Answer from the drawing. Dimensions are ordinates in mm from the lowest x, y and z of the part. Round coordinates to 2 decimals unless told otherwise and drop trailing zeros. Write each loop counter-clockwise with the first axis right and the second up, starting at its lowest first coordinate (ties: lowest second). Pieces come first, ordered by that corner, then holes. Notation, with made-up numbers: M 37.25,10.5 L 81.25,10.5 A27 cw 81.25,28.5 Z; hole C 68.5,43 d5. An arc over 180 degrees is marked long. One line per item, written item: value. Start each with the question number.
(1) Section C-C (z = 1.95) is taken. Determine the outline of the cut face in (x, y).
(2) Section D-D (x = 82.45) is taken. Determine the outline of the cut face in (y, z).
(3) Section A-A (y = 37.5) is taken. Determine the outline of the cut face in (x, z).
(4) Consider probe 1 along Y at (x, z) = (58, 0.8); probe 2 along X at (y, z) = (22, 5.25); probe 3 along Y at (x, z) = (82.45, 1.85). Determine where each line is inside the solid, lowest interval first.
(5) Given P1, Ø3, axis at x = 8.5, z = 2, coming from the -Y side; P2, Ø1.8, axis at x = 13, z = 2, coming from the +Y side, each flat-ended and moving along its own axis, determine where each tip first touches the part or whether it passes through.
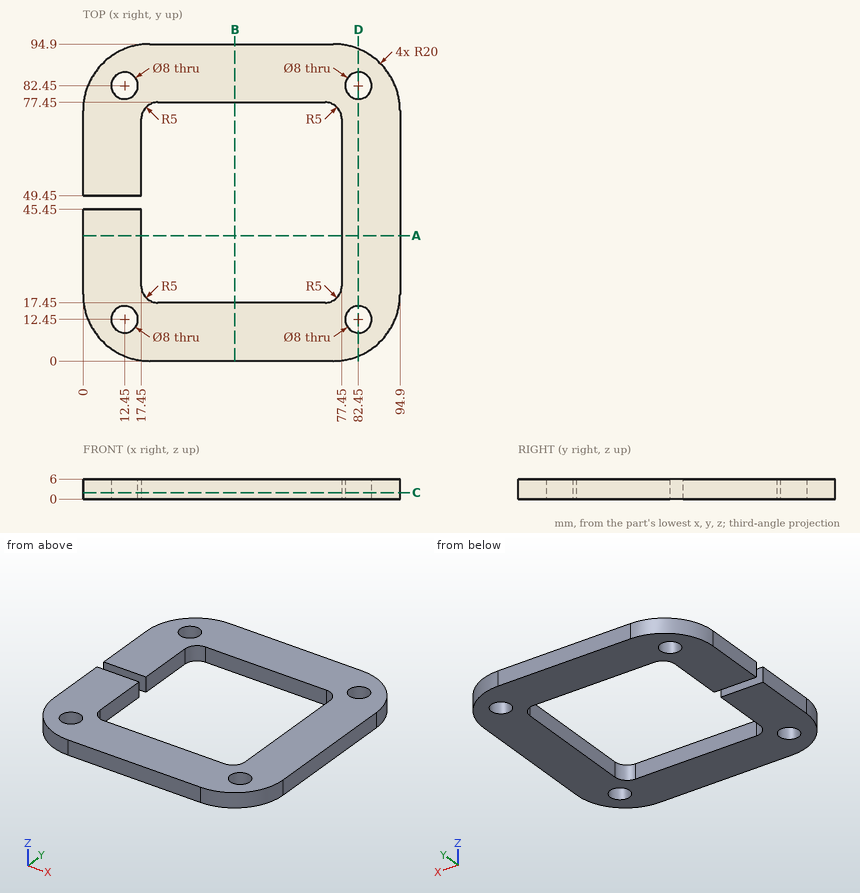
Recorded:
1. outline: M 0,20 A20 ccw 20,0 L 74.9,0 A20 ccw 94.9,20 L 94.9,74.9 A20 ccw 74.9,94.9 L 20,94.9 A20 ccw 0,74.9 L 0,49.45 L 17.45,49.45 L 17.45,72.45 A5 cw 22.45,77.45 L 72.45,77.45 A5 cw 77.45,72.45 L 77.45,22.45 A5 cw 72.45,17.45 L 22.45,17.45 A5 cw 17.45,22.45 L 17.45,45.45 L 0,45.45 Z; hole C 12.45,12.45 d8; hole C 12.45,82.45 d8; hole C 82.45,12.45 d8; hole C 82.45,82.45 d8
2. outline: M 1.48,0 L 8.45,0 L 8.45,6 L 1.48,6 Z; M 16.45,0 L 78.45,0 L 78.45,6 L 16.45,6 Z; M 86.45,0 L 93.42,0 L 93.42,6 L 86.45,6 Z
3. outline: M 0,0 L 17.45,0 L 17.45,6 L 0,6 Z; M 77.45,0 L 94.9,0 L 94.9,6 L 77.45,6 Z
4. probe 1: y = 0 to 17.45, 77.45 to 94.9
4. probe 2: x = 0 to 17.47, 77.43 to 94.9
4. probe 3: y = 1.48 to 8.45, 16.45 to 78.45, 86.45 to 93.42
5. P1: stops at y = 2.68
5. P2: stops at y = 93.95
